```python
from build123d import *

# Parameters (mm, degrees)
SKIZZE1_R                            = 5
ZYLINDER_DEPTH                       = 2.2
SCHNITT_LINEAR_AUSTRAGEN1_DEPTH      = 10
SCHNITT_LINEAR_AUSTRAGEN1_DEPTH_BACK = 5
SKIZZE4_R                            = 4.5
SKIZZE6_R                            = 22.5
FASSUNG_OBJEKTTR_GERGEWINDE_DEPTH    = 7
SKIZZE11_R                           = 20.3
BOHRUNG_F_R_INNENGEWINDE_DEPTH       = 6
SKIZZE13_R                           = 8
ZYLINDER_F_R_GEWINDE_DEPTH           = 3
SKIZZE16_R                           = 2.6
LINSENEINSATZ_DEPTH                  = 10
GEWINDE1_PITCH                       = 1.5
SKIZZE17_W                           = 26.5
SKIZZE17_H                           = 49.541135346
SCHLITZ_F_R_SLIDE_DEPTH              = 1.6
SKIZZE21_R                           = 6.5
FILTEREINSATZ_DEPTH                  = 2.5


with BuildPart() as part:
    # Skizze1 → Zylinder (new body)
    with BuildSketch(Plane(origin=(0, 0, 0), x_dir=(1, 0, 0), z_dir=(0, 1, 0))):
        with Locations(Location((-18.043745097, 0, 0), (0, 0, 270))):
            Circle(SKIZZE1_R)
    extrude(amount=ZYLINDER_DEPTH)

    # Skizze4 → Schnitt-Linear austragen1 (cut, two sides: drawn at the far end of the back side and taken through both)
    with BuildSketch(Plane(origin=(0, 2.2, 0), x_dir=(1, 0, 0), z_dir=(0, 1, 0)).offset(-SCHNITT_LINEAR_AUSTRAGEN1_DEPTH_BACK)):
        with Locations(Location((-18.043745097, 0, 0), (0, 0, 270))):
            Circle(SKIZZE4_R)
    extrude(amount=SCHNITT_LINEAR_AUSTRAGEN1_DEPTH + SCHNITT_LINEAR_AUSTRAGEN1_DEPTH_BACK, mode=Mode.SUBTRACT)

    # Skizze6 → Fassung Objektträgergewinde (add)
    with BuildSketch(Plane(origin=(0, 0, 0), x_dir=(-1, 0, 0), z_dir=(0, -1, 0))):
        with Locations(Location((18.043745097, 0, 0), (0, 0, 90))):
            Circle(SKIZZE6_R)
    extrude(amount=FASSUNG_OBJEKTTR_GERGEWINDE_DEPTH)

    # Skizze11 → Bohrung für Innengewinde (cut)
    with BuildSketch(Plane(origin=(0, -7, 0), x_dir=(-1, 0, 0), z_dir=(0, -1, 0))):
        with Locations(Location((18.043745097, 0, 0), (0, 0, 90))):
            Circle(SKIZZE11_R)
    extrude(amount=-BOHRUNG_F_R_INNENGEWINDE_DEPTH, mode=Mode.SUBTRACT)

    # Skizze13 → Zylinder für Gewinde (add)
    with BuildSketch(Plane(origin=(0, 0, 0), x_dir=(-1, 0, 0), z_dir=(0, -1, 0))):
        with Locations(Location((18.043745097, 0, 0), (0, 0, 90))):
            Circle(SKIZZE13_R)
    extrude(amount=-ZYLINDER_F_R_GEWINDE_DEPTH)

    # Skizze16 → Linseneinsatz (cut)
    with BuildSketch(Plane(origin=(0, -7, 0), x_dir=(-1, 0, 0), z_dir=(0, -1, 0))):
        with Locations(Location((18.043745097, 0, 0), (0, 0, 90))):
            Circle(SKIZZE16_R)
    extrude(amount=-LINSENEINSATZ_DEPTH, mode=Mode.SUBTRACT)

    # Gewinde1: the profile of Gewindeprofil1 profile screwed along a right-hand helix of 2.333333 turns, 8 arcs to a turn; built about Z, then put on its axis
    gewinde1_z = Axis((0, 0, 0), (0, 0, 1))
    gewinde1_corners = [(8.0003, 0, -0.000173205), (8.0003, 0, 1.312673201), (7.188101187, 0, 0.843749998), (7.188101187, 0, 0.468749998)]
    with BuildLine(mode=Mode.PRIVATE) as gewinde1_profile:
        Line(gewinde1_corners[0], gewinde1_corners[1])
        Line(gewinde1_corners[1], gewinde1_corners[2])
        Line(gewinde1_corners[2], gewinde1_corners[3])
        Line(gewinde1_corners[3], gewinde1_corners[0])
    gewinde1_cap = Face(gewinde1_profile.wire())
    gewinde1_turn_angles = [0, 22.5, 45, 67.5, 90, 112.5, 135, 157.5, 180, 202.5, 225, 247.5, 270, 292.5, 315, 337.5, 360]
    gewinde1_turn_weights = [1, 0.9238795325112867, 1, 0.9238795325112867, 1, 0.9238795325112867, 1, 0.9238795325112867, 1, 0.9238795325112867, 1, 0.9238795325112867, 1, 0.9238795325112867, 1, 0.9238795325112867, 1]
    gewinde1_turn_rails = [Edge.make_bspline([Vector(p[0], p[1], 0).rotate(gewinde1_z, gewinde1_turn_angles[k]) / gewinde1_turn_weights[k] + Vector(0, 0, p[2] + GEWINDE1_PITCH * gewinde1_turn_angles[k] / 360) for k in range(17)], [0, 0, 0, 1, 1, 2, 2, 3, 3, 4, 4, 5, 5, 6, 6, 7, 7, 8, 8, 8], 2, gewinde1_turn_weights) for p in gewinde1_corners]
    gewinde1_turn_sides = [Face.make_surface_from_curves(gewinde1_turn_rails[p[0]], gewinde1_turn_rails[p[1]]) for p in [(0, 1), (1, 2), (2, 3), (3, 0)]]
    gewinde1_last_angles = [720, 742.5, 765, 787.5, 810, 825, 840]
    gewinde1_last_weights = [1, 0.9238795325112867, 1, 0.9238795325112867, 1, 0.9659258262890685, 1]
    gewinde1_last_rails = [Edge.make_bspline([Vector(p[0], p[1], 0).rotate(gewinde1_z, gewinde1_last_angles[k]) / gewinde1_last_weights[k] + Vector(0, 0, p[2] + GEWINDE1_PITCH * gewinde1_last_angles[k] / 360) for k in range(7)], [0, 0, 0, 1, 1, 2, 2, 3, 3, 3], 2, gewinde1_last_weights) for p in gewinde1_corners]
    gewinde1_last_sides = [Face.make_surface_from_curves(gewinde1_last_rails[p[0]], gewinde1_last_rails[p[1]]) for p in [(0, 1), (1, 2), (2, 3), (3, 0)]]
    gewinde1 = Plane(origin=(-18.043745097, 4.6, 0), x_dir=(-1, 0, 0), z_dir=(0, -1, 0)) * Solid(Shell([*[p.moved(Location((0, 0, GEWINDE1_PITCH * i))) for i in range(2) for p in gewinde1_turn_sides], *gewinde1_last_sides, gewinde1_cap, gewinde1_cap.rotate(gewinde1_z, 840).moved(Location((0, 0, GEWINDE1_PITCH * 840 / 360)))]))
    add(gewinde1, mode=Mode.SUBTRACT)

    # Skizze17 → Schlitz für Slide (cut)
    with BuildSketch(Plane(origin=(0, -2, 0), x_dir=(1, 0, 0), z_dir=(0, 1, 0))):
        with Locations((-18.043745097, 0)):
            Rectangle(SKIZZE17_W, SKIZZE17_H)
    extrude(amount=-SCHLITZ_F_R_SLIDE_DEPTH, mode=Mode.SUBTRACT)

    # Skizze21 → Filtereinsatz (cut)
    with BuildSketch(Plane(origin=(0, -1, 0), x_dir=(-1, 0, 0), z_dir=(0, -1, 0))):
        with Locations(Location((18.043745097, 0, 0), (0, 0, 90))):
            Circle(SKIZZE21_R)
    extrude(amount=-FILTEREINSATZ_DEPTH, mode=Mode.SUBTRACT)


solid = part.part
```
Geometry: final body of the model. Coordinates: model frame, mm. A direction names the side the tool comes from. Round coordinates to 2 decimals unless told otherwise and drop trailing zeros. Write each loop counter-clockwise with the first axis right and the second up, starting at its lowest first coordinate (ties: lowest second). Pieces come first, ordered by that corner, then holes. Notation, with made-up numbers: (54, 19) -> (107, 19) arc R34 cw to (107, 58) -> close; hole circle Ø9 at (28, 65.25). An arc over 180 degrees is marked (long way). Return JSON: item names as keys, results as strings.
Q1. Section A-A on y = -3. Return the cut outline in (x, z).
From the geometry:
{"outline": "(-31.29, -18.18) -> (-31.29, -15.38) arc R20.3 cw to (-31.29, 15.38) -> (-31.29, 18.18) arc R22.5 ccw to start; (-4.79, -18.18) arc R22.5 ccw to (-4.79, 18.18) -> (-4.79, 15.38) arc R20.3 cw to (-4.79, -15.38) -> close"}
Q2. First-contact query: pin 1 Ø1.5 at (x, z) = (-17, -17.5) entering from -Y; pin 2 Ø6 at (x, z) = (-28.5, 14.5) entering from +Y; pin 3 Ø10.5 at (x, z) = (-18.04, 0) entering from -Y; pin 4 Ø4.5 at (x, z) = (-18.04, 0) entering from +Y. Flat tips, straight axial feed; report the tip coordinate or a pass-through.
From the geometry:
{"pin 1": "y = -1", "pin 2": "y = 0", "pin 3": "y = 1.5", "pin 4": "through"}
Q3. Section B-B on x = -6.5. Return the cut outline in (y, z), and give its area (3 significant figures).
From the geometry:
{"outline": "(-7, -19.31) -> (-3.6, -19.31) -> (-3.6, -16.7) -> (-7, -16.7) -> close; (-7, 16.7) -> (-3.6, 16.7) -> (-3.6, 19.31) -> (-7, 19.31) -> close; (-2, -19.31) -> (0, -19.31) -> (0, 19.31) -> (-2, 19.31) -> (-2, 16.7) -> (-1, 16.7) -> (-1, -16.7) -> (-2, -16.7) -> close", "area": "61.6 mm2"}
Q4. Section D-D on x = -32.5. Return the cut outline in (y, z), and give its area (3 significant figures).
From the geometry:
{"outline": "(-7, -17.24) -> (0, -17.24) -> (0, 17.24) -> (-7, 17.24) -> (-7, 14.25) -> (-1, 14.25) -> (-1, -14.25) -> (-7, -14.25) -> close", "area": "70.4 mm2"}
Q5. Ray query, line 1 (Y direction, x = -29, z = 19); line 2 (X direction, y = -0.05, z = 0); line 3 (Y direction, x = -26, z = 10). Return the intervals inside material, ascending.
From the geometry:
{"line 1": "-7 to -3.6, -2 to 0", "line 2": "-40.54 to -24.54, -11.54 to 4.46", "line 3": "-1 to 0"}
Q6. Section C-C on z = 19. Return the cut outline in (x, y).
From the geometry:
{"outline": "(-30.1, -7) -> (-25.19, -7) -> (-25.19, -3.6) -> (-30.1, -3.6) -> close; (-30.1, -2) -> (-25.19, -2) -> (-25.19, -1) -> (-10.9, -1) -> (-10.9, -2) -> (-5.99, -2) -> (-5.99, 0) -> (-30.1, 0) -> close; (-10.9, -7) -> (-5.99, -7) -> (-5.99, -3.6) -> (-10.9, -3.6) -> close"}
Q7. Set-up query: faces 1 (the flat face through (-19, -3.6, 21)), 2 (the flat face through (-20, 3, -2)), 3 (the cylindrical face through (-11.6, 0.23, 0.85)). Return all of +Z, -Z, +X, -X, +Y, -Y with unobstructed straight access to the full face (end or side cutting, diameter ignored); none if empty.
From the geometry:
{"face 1": "+Z, -Z", "face 2": "+Z, -Z, +X, -X, +Y", "face 3": "-Y"}
Q8. Mould query, pull axis Y, two halves, no side actions, for faces 4 (the flat face through (-17, -2, -21)), 5 (the flat face through (-1, -7, 12)), 6 (the flat face through (-19, -2, 21)), 7 (the flat face through (-28, 0, 0)). Classes: +Y half, -Y half, draft (parallel to the pull), parting line (faces both ways), or undercut.
From the geometry:
{"face 4": "undercut", "face 5": "-Y half", "face 6": "undercut", "face 7": "+Y half"}
